from build123d import *

# Parameters (mm, degrees)
BOSS_EXTRUDE1_DEPTH                           = 1.5875
CSK_FOR_6_FLAT_HEAD_SOCKET_CAP_SCREW1_A_COUNT = 2
CSK_FOR_6_FLAT_HEAD_SOCKET_CAP_SCREW1_A_PITCH = 31.75
CSK_FOR_6_FLAT_HEAD_SOCKET_CAP_SCRE_2_COUNT   = 2
CSK_FOR_6_FLAT_HEAD_SOCKET_CAP_SCRE_2_PITCH   = 63.5
CSK_FOR_6_FLAT_HEAD_SOCKET_CAP_SCRE_3_COUNT   = 2
CSK_FOR_6_FLAT_HEAD_SOCKET_CAP_SCRE_3_PITCH   = 95.25
CSK_FOR_6_FLAT_HEAD_SOCKET_CAP_SCRE_4_COUNT   = 2
CSK_FOR_6_FLAT_HEAD_SOCKET_CAP_SCRE_4_PITCH   = 127
CSK_FOR_6_FLAT_HEAD_SOCKET_CAP_SCRE_5_COUNT   = 2
CSK_FOR_6_FLAT_HEAD_SOCKET_CAP_SCRE_5_PITCH   = 158.75
CSK_FOR_6_FLAT_HEAD_SOCKET_CAP_SCRE_6_COUNT   = 2
CSK_FOR_6_FLAT_HEAD_SOCKET_CAP_SCRE_6_PITCH   = 190.5
CSK_FOR_6_FLAT_HEAD_SOCKET_CAP_SCRE_7_COUNT   = 2
CSK_FOR_6_FLAT_HEAD_SOCKET_CAP_SCRE_7_PITCH   = 222.25
CSK_FOR_6_FLAT_HEAD_SOCKET_CAP_SCRE_8_COUNT   = 2
CSK_FOR_6_FLAT_HEAD_SOCKET_CAP_SCRE_8_PITCH   = 254
CSK_FOR_6_FLAT_HEAD_SOCKET_CAP_SCRE_9_COUNT   = 2
CSK_FOR_6_FLAT_HEAD_SOCKET_CAP_SCRE_9_PITCH   = 285.75
CSK_FOR_6_FLAT_HEAD_SOCKET_CAP_SCRE_10_COUNT  = 2
CSK_FOR_6_FLAT_HEAD_SOCKET_CAP_SCRE_10_PITCH  = 317.5
CSK_FOR_6_FLAT_HEAD_SOCKET_CAP_SCREW2_A_COUNT = 2
CSK_FOR_6_FLAT_HEAD_SOCKET_CAP_SCREW2_A_PITCH = 15.24
CSK_FOR_6_FLAT_HEAD_SOCKET_CAP_SCRE_11_COUNT  = 2
CSK_FOR_6_FLAT_HEAD_SOCKET_CAP_SCRE_11_PITCH  = 30.48
CSK_FOR_6_FLAT_HEAD_SOCKET_CAP_SCRE_12_COUNT  = 2
CSK_FOR_6_FLAT_HEAD_SOCKET_CAP_SCRE_12_PITCH  = 45.72
CSK_FOR_6_FLAT_HEAD_SOCKET_CAP_SCRE_13_COUNT  = 2
CSK_FOR_6_FLAT_HEAD_SOCKET_CAP_SCRE_13_PITCH  = 60.96
CSK_FOR_6_FLAT_HEAD_SOCKET_CAP_SCRE_14_COUNT  = 2
CSK_FOR_6_FLAT_HEAD_SOCKET_CAP_SCRE_14_PITCH  = 76.2
CSK_FOR_6_FLAT_HEAD_SOCKET_CAP_SCRE_15_COUNT  = 2
CSK_FOR_6_FLAT_HEAD_SOCKET_CAP_SCRE_15_PITCH  = 91.44


with BuildPart() as part:
    # Sketch1 → Boss-Extrude1 (new body)
    with BuildSketch(Plane.XY):
        with BuildLine():
            Line((0, 15.875), (404.9268, 139.5476))
            Line((404.9268, 139.5476), (430.3268, 139.5476))
            Line((430.3268, 139.5476), (430.3268, 15.875))
            Line((430.3268, 15.875), (370.0018, 15.875))
            ThreePointArc((370.0018, 15.875), (365.511671939, 14.015128061), (363.6518, 9.525))
            Line((363.6518, 9.525), (363.6518, 6.35))
            ThreePointArc((363.6518, 6.35), (361.791928061, 1.859871939), (357.3018, 0))
            Line((357.3018, 0), (6.35, 0))
            ThreePointArc((6.35, 0), (1.859871939, 1.859871939), (0, 6.35))
            Line((0, 6.35), (0, 15.875))
        make_face()
    extrude(amount=BOSS_EXTRUDE1_DEPTH)

    # Sketch3 → CSK for #6 Flat Head Socket Cap Screw1 (revolve, cut)
    with BuildSketch(Plane(origin=(343.3318, 7.9375, 1.5875), x_dir=(0, -1, 0), z_dir=(1, 0, 0))):
        Polygon((0, 0), (0, 2.6228539), (1.8288, 1.524), (1.8288, 1.504796913), (3.1369, 0), align=None)
    csk_for_6_flat_head_socket_cap_screw1 = revolve(axis=Axis((343.3318, 7.9375, 7.9375), (0, 0, -1)), mode=Mode.SUBTRACT)

    # CSK for #6 Flat Head Socket Cap Screw1 a: CSK for #6 Flat Head Socket Cap Screw1 ×2
    with Locations(*[(-i * CSK_FOR_6_FLAT_HEAD_SOCKET_CAP_SCREW1_A_PITCH, 0, 0) for i in range(1, CSK_FOR_6_FLAT_HEAD_SOCKET_CAP_SCREW1_A_COUNT)]):
        add(csk_for_6_flat_head_socket_cap_screw1, mode=Mode.SUBTRACT)

    # CSK for _6 Flat Head Socket Cap Scre 2: CSK for #6 Flat Head Socket Cap Screw1 ×2
    with Locations(*[(-i * CSK_FOR_6_FLAT_HEAD_SOCKET_CAP_SCRE_2_PITCH, 0, 0) for i in range(1, CSK_FOR_6_FLAT_HEAD_SOCKET_CAP_SCRE_2_COUNT)]):
        add(csk_for_6_flat_head_socket_cap_screw1, mode=Mode.SUBTRACT)

    # CSK for _6 Flat Head Socket Cap Scre 3: CSK for #6 Flat Head Socket Cap Screw1 ×2
    with Locations(*[(-i * CSK_FOR_6_FLAT_HEAD_SOCKET_CAP_SCRE_3_PITCH, 0, 0) for i in range(1, CSK_FOR_6_FLAT_HEAD_SOCKET_CAP_SCRE_3_COUNT)]):
        add(csk_for_6_flat_head_socket_cap_screw1, mode=Mode.SUBTRACT)

    # CSK for _6 Flat Head Socket Cap Scre 4: CSK for #6 Flat Head Socket Cap Screw1 ×2
    with Locations(*[(-i * CSK_FOR_6_FLAT_HEAD_SOCKET_CAP_SCRE_4_PITCH, 0, 0) for i in range(1, CSK_FOR_6_FLAT_HEAD_SOCKET_CAP_SCRE_4_COUNT)]):
        add(csk_for_6_flat_head_socket_cap_screw1, mode=Mode.SUBTRACT)

    # CSK for _6 Flat Head Socket Cap Scre 5: CSK for #6 Flat Head Socket Cap Screw1 ×2
    with Locations(*[(-i * CSK_FOR_6_FLAT_HEAD_SOCKET_CAP_SCRE_5_PITCH, 0, 0) for i in range(1, CSK_FOR_6_FLAT_HEAD_SOCKET_CAP_SCRE_5_COUNT)]):
        add(csk_for_6_flat_head_socket_cap_screw1, mode=Mode.SUBTRACT)

    # CSK for _6 Flat Head Socket Cap Scre 6: CSK for #6 Flat Head Socket Cap Screw1 ×2
    with Locations(*[(-i * CSK_FOR_6_FLAT_HEAD_SOCKET_CAP_SCRE_6_PITCH, 0, 0) for i in range(1, CSK_FOR_6_FLAT_HEAD_SOCKET_CAP_SCRE_6_COUNT)]):
        add(csk_for_6_flat_head_socket_cap_screw1, mode=Mode.SUBTRACT)

    # CSK for _6 Flat Head Socket Cap Scre 7: CSK for #6 Flat Head Socket Cap Screw1 ×2
    with Locations(*[(-i * CSK_FOR_6_FLAT_HEAD_SOCKET_CAP_SCRE_7_PITCH, 0, 0) for i in range(1, CSK_FOR_6_FLAT_HEAD_SOCKET_CAP_SCRE_7_COUNT)]):
        add(csk_for_6_flat_head_socket_cap_screw1, mode=Mode.SUBTRACT)

    # CSK for _6 Flat Head Socket Cap Scre 8: CSK for #6 Flat Head Socket Cap Screw1 ×2
    with Locations(*[(-i * CSK_FOR_6_FLAT_HEAD_SOCKET_CAP_SCRE_8_PITCH, 0, 0) for i in range(1, CSK_FOR_6_FLAT_HEAD_SOCKET_CAP_SCRE_8_COUNT)]):
        add(csk_for_6_flat_head_socket_cap_screw1, mode=Mode.SUBTRACT)

    # CSK for _6 Flat Head Socket Cap Scre 9: CSK for #6 Flat Head Socket Cap Screw1 ×2
    with Locations(*[(-i * CSK_FOR_6_FLAT_HEAD_SOCKET_CAP_SCRE_9_PITCH, 0, 0) for i in range(1, CSK_FOR_6_FLAT_HEAD_SOCKET_CAP_SCRE_9_COUNT)]):
        add(csk_for_6_flat_head_socket_cap_screw1, mode=Mode.SUBTRACT)

    # CSK for _6 Flat Head Socket Cap Scre 10: CSK for #6 Flat Head Socket Cap Screw1 ×2
    with Locations(*[(-i * CSK_FOR_6_FLAT_HEAD_SOCKET_CAP_SCRE_10_PITCH, 0, 0) for i in range(1, CSK_FOR_6_FLAT_HEAD_SOCKET_CAP_SCRE_10_COUNT)]):
        add(csk_for_6_flat_head_socket_cap_screw1, mode=Mode.SUBTRACT)

    # Sketch5 → CSK for #6 Flat Head Socket Cap Screw2 (revolve, cut)
    with BuildSketch(Plane(origin=(417.6268, 123.4313, 1.5875), x_dir=(0, -1, 0), z_dir=(1, 0, 0))):
        Polygon((0, 0), (0, 2.6228539), (1.8288, 1.524), (1.8288, 1.504796913), (3.1369, 0), align=None)
    csk_for_6_flat_head_socket_cap_screw2 = revolve(axis=Axis((417.6268, 123.4313, 7.9375), (0, 0, -1)), mode=Mode.SUBTRACT)

    # CSK for #6 Flat Head Socket Cap Screw2 a: CSK for #6 Flat Head Socket Cap Screw2 ×2
    with Locations(*[(0, -i * CSK_FOR_6_FLAT_HEAD_SOCKET_CAP_SCREW2_A_PITCH, 0) for i in range(1, CSK_FOR_6_FLAT_HEAD_SOCKET_CAP_SCREW2_A_COUNT)]):
        add(csk_for_6_flat_head_socket_cap_screw2, mode=Mode.SUBTRACT)

    # CSK for _6 Flat Head Socket Cap Scre 11: CSK for #6 Flat Head Socket Cap Screw2 ×2
    with Locations(*[(0, -i * CSK_FOR_6_FLAT_HEAD_SOCKET_CAP_SCRE_11_PITCH, 0) for i in range(1, CSK_FOR_6_FLAT_HEAD_SOCKET_CAP_SCRE_11_COUNT)]):
        add(csk_for_6_flat_head_socket_cap_screw2, mode=Mode.SUBTRACT)

    # CSK for _6 Flat Head Socket Cap Scre 12: CSK for #6 Flat Head Socket Cap Screw2 ×2
    with Locations(*[(0, -i * CSK_FOR_6_FLAT_HEAD_SOCKET_CAP_SCRE_12_PITCH, 0) for i in range(1, CSK_FOR_6_FLAT_HEAD_SOCKET_CAP_SCRE_12_COUNT)]):
        add(csk_for_6_flat_head_socket_cap_screw2, mode=Mode.SUBTRACT)

    # CSK for _6 Flat Head Socket Cap Scre 13: CSK for #6 Flat Head Socket Cap Screw2 ×2
    with Locations(*[(0, -i * CSK_FOR_6_FLAT_HEAD_SOCKET_CAP_SCRE_13_PITCH, 0) for i in range(1, CSK_FOR_6_FLAT_HEAD_SOCKET_CAP_SCRE_13_COUNT)]):
        add(csk_for_6_flat_head_socket_cap_screw2, mode=Mode.SUBTRACT)

    # CSK for _6 Flat Head Socket Cap Scre 14: CSK for #6 Flat Head Socket Cap Screw2 ×2
    with Locations(*[(0, -i * CSK_FOR_6_FLAT_HEAD_SOCKET_CAP_SCRE_14_PITCH, 0) for i in range(1, CSK_FOR_6_FLAT_HEAD_SOCKET_CAP_SCRE_14_COUNT)]):
        add(csk_for_6_flat_head_socket_cap_screw2, mode=Mode.SUBTRACT)

    # CSK for _6 Flat Head Socket Cap Scre 15: CSK for #6 Flat Head Socket Cap Screw2 ×2
    with Locations(*[(0, -i * CSK_FOR_6_FLAT_HEAD_SOCKET_CAP_SCRE_15_PITCH, 0) for i in range(1, CSK_FOR_6_FLAT_HEAD_SOCKET_CAP_SCRE_15_COUNT)]):
        add(csk_for_6_flat_head_socket_cap_screw2, mode=Mode.SUBTRACT)


solid = part.part
The listing builds one solid part. Answer for the finished solid, in the listing's coordinates (mm). Give positions to 0.01 mm unless a question says otherwise; leave off trailing zeros. Order: outer loops, then holes, each group sorted by start corner. A loop starts at its lowest first (then second) coordinate and runs counter-clockwise, first axis right, second up. Notation, with made-up numbers: (23.5, 49) - (82.5, 49) arc R32 cw to (82.5, 77) - close; hole circle Ø11 at (-29, 51.5). An arc over 180 degrees is marked (long way). One line per item, written item: value. Start each with the question number.
1) Given pin 1 Ø6 at (x, y) = (417.63, 47.23) entering from +Z; pin 2 Ø5 at (x, y) = (248.08, 7.94) entering from +Z, each flat-ended and moving along its own axis, determine where each tip first touches the part or whether it passes through.
2) A cutting plane is placed at B-B on x = 272. Give the vertices of the cut face in (y, z), then the cut area to 3 significant figures.
3) A cutting plane is placed at A-A on z = 0.55. State how many separate pieces and enclosed holes the cut face has, then the cut area to 3 significant figures.
4) A cutting plane is placed at C-C on y = 20. Give the vertices of the cut face in (x, z).
5) Find the intervals of material crossed by L1, parallel to Y at x = 24.5, z = 1.25; L2, parallel to Y at x = 33, z = 0.4; L3, parallel to Y at x = 194, z = 1.4, in increasing order.
Answer sheet:
1. pin 1: stops at z = 1.43
1. pin 2: stops at z = 0.86
2. outline: (0, 0) - (98.95, 0) - (98.95, 1.59) - (0, 1.59) - close
2. area: 157 mm2
3. separate pieces: 1
3. enclosed holes: 18
3. area: 33,700 mm2
4. outline: (13.51, 0) - (430.33, 0) - (430.33, 1.59) - (13.51, 1.59) - close
5. L1: y = 0 to 5.43, 10.45 to 23.36
5. L2: y = 0 to 25.95
5. L3: y = 0 to 75.13
